Work out the finished part from the listing and answer in its coordinate system (mm). Give positions to 0.01 mm unless a question says otherwise; leave off trailing zeros. Order: outer loops, then holes, each group sorted by start corner. A loop starts at its lowest first (then second) coordinate and runs counter-clockwise, first axis right, second up.
```python
from build123d import *

# Parameters (mm, degrees)
F0_R     = 5.7735026919
F0_R_2   = 3
F1_DEPTH = 2
F3_R     = 0.8
F2_R     = 6
F4_DEPTH = 4.001


with BuildPart() as f1:
    # F0 (on Front) → F1 (new body, symmetric)
    with BuildSketch(Plane.XZ):
        Circle(F0_R)
        Circle(F0_R_2, mode=Mode.SUBTRACT)
    extrude(amount=F1_DEPTH, both=True)

    # F3
    f3_edges = [f1.edges().sort_by_distance(p)[0] for p in [
        (-5.773503, -2, 0),
        (-5.773503, 2, 0),
    ]]
    fillet(f3_edges, radius=F3_R)

    # F2 (on face) → F4 (cut, through all)
    with BuildSketch(Plane.XZ.offset(2)):
        Circle(F2_R)
        Polygon((0, -5.7735026919), (-5, -2.8867513459), (-5, 2.8867513459), (0, 5.7735026919), (5, 2.8867513459), (5, -2.8867513459), align=None, mode=Mode.SUBTRACT)
    extrude(amount=-F4_DEPTH, mode=Mode.SUBTRACT)


solid = f1.part
```
1. The part is cut by section B-B (y = -0.25). Write down the section's boundary in (x, z).
Findings below:
outline: (-5, -2.89) - (0, -5.77) - (5, -2.89) - (5, 2.89) - (0, 5.77) - (-5, 2.89) - close; hole circle Ø6 at (0, 0)
2. Given P1, Ø1, axis at x = -1, y = -1, coming from the -Z side; P2, Ø3.5, axis at x = 0, z = 0, coming from the +Y side; P3, Ø2, axis at y = 1, z = 3, coming from the +X side, each flat-ended and moving along its own axis, determine where each tip first touches the part or whether it passes through.
Findings below:
P1: stops at z = -5.48
P2: passes through
P3: stops at x = 5
3. The mould has two halves that part along X. Classify faces 1 (the face through (-3, 0, 0)), 2 (the face through (-0.1, -2, -3.2)), 3 (the face through (-2.465, -0.028, -4.35)): pulls with the +X half, pulls with the -X half, needs draft (parallel to the pull), parting line crosses it, or undercut.
Findings below:
face 1: undercut
face 2: needs draft
face 3: pulls with the -X half
4. Straight lines are drawn through the part: probe 1 along Z at (x, y) = (-2, 0.25); probe 2 along X at (y, z) = (1.8, -0.25); probe 3 along Z at (x, y) = (2.5, 1.1). For each, find the intervals that lie inside material, in ascending order.
Findings below:
probe 1: z = -4.62 to -2.24, 2.24 to 4.62
probe 2: x = -5 to -2.99, 2.99 to 5
probe 3: z = -4.33 to -1.66, 1.66 to 4.33
